Read the model definition and answer for the solid it produces. Units are mm, in the model's axes. A direction names the side the tool comes from. Round coordinates to 2 decimals unless told otherwise and drop trailing zeros. Loops run counter-clockwise (first coordinate to the right, second up) from the corner with the lowest first, then second, coordinate; pieces in that order, holes last. Notation, with made-up numbers: (-16.75, 33) -> (11.25, 33) arc R20 ccw to (11.25, 62) -> close; hole circle Ø5 at (-15, -7.5). An arc over 180 degrees is marked (long way). Put each result on its own line as item: value.
from build123d import *

# Parameters (mm, degrees)
SKETCH_R        = 14
SKETCH_R_2      = 8
PAD_DEPTH       = 2
SKETCH001_R     = 10
SKETCH001_R_2   = 8
PAD001_DEPTH    = 22
CHAMFER_SIZE    = 0.5
CHAMFER001_SIZE = 0.5
CHAMFER002_SIZE = 0.5
CHAMFER003_SIZE = 1


with BuildPart() as part:
    # Sketch → Pad (new body)
    with BuildSketch(Plane.XY):
        Circle(SKETCH_R)
        Circle(SKETCH_R_2, mode=Mode.SUBTRACT)
    extrude(amount=PAD_DEPTH)

    # Sketch001 (on Face4 of Pad) → Pad001 (join)
    with BuildSketch(Plane.XY.offset(2)):
        Circle(SKETCH001_R)
        Circle(SKETCH001_R_2, mode=Mode.SUBTRACT)
    extrude(amount=PAD001_DEPTH)

    # Chamfer
    chamfer_edges = [part.edges().sort_by_distance(p)[0] for p in [
        (-8, 0, 24),
    ]]
    chamfer(chamfer_edges, length=CHAMFER_SIZE)

    # Chamfer001
    chamfer001_edges = [part.edges().sort_by_distance(p)[0] for p in [
        (-10, 0, 24),
    ]]
    chamfer(chamfer001_edges, length=CHAMFER001_SIZE)

    # Chamfer002
    chamfer002_edges = [part.edges().sort_by_distance(p)[0] for p in [
        (-8, 0, 0),
    ]]
    chamfer(chamfer002_edges, length=CHAMFER002_SIZE)

    # Chamfer003
    chamfer003_edges = [part.edges().sort_by_distance(p)[0] for p in [
        (-14, 0, 2),
    ]]
    chamfer(chamfer003_edges, length=CHAMFER003_SIZE)


solid = part.part
Item 1: Flat-ended cylindrical pins translate along their axes: pin 1 Ø4 at (y, z) = (4.5, 21.5) entering from +X; pin 2 Ø4 at (x, z) = (-6, 6) entering from -Y; pin 3 Ø1.5 at (y, z) = (-3.5, 11.5) entering from -X. Find the tip coordinate at first contact, or state that the pin passes through.
Derived:
pin 1: stops at x = 9.68
pin 2: stops at y = -9.17
pin 3: stops at x = -9.61
Item 2: The part is cut by section A-A (x = 0). Determine the outline of the cut face in (y, z), then the cut area to 3 significant figures.
Derived:
outline: (-14, 0) -> (-8.5, 0) -> (-8, 0.5) -> (-8, 23.5) -> (-8.5, 24) -> (-9.5, 24) -> (-10, 23.5) -> (-10, 2) -> (-13, 2) -> (-14, 1) -> close; (8, 0.5) -> (8.5, 0) -> (14, 0) -> (14, 1) -> (13, 2) -> (10, 2) -> (10, 23.5) -> (9.5, 24) -> (8.5, 24) -> (8, 23.5) -> close
area: 110 mm^2
Item 3: Which of the six approach directions +Z, -Z, +X, -X, +Y, -Y give full straight-line access (tool end or side, diameter ignored) to faces 4 (the cylindrical face through (-2.17, -9.76, 12.6)), 5 (the flat face through (0, -9, 0))?
Derived:
face 4: +Z
face 5: -Z, +X, -X, +Y, -Y
Item 4: For a pull along Y with two mould halves and no side action, classify faces 1 (the cylindrical face through (12.932, -5.362, 0.493)), 2 (the flat face through (7, -8, 2)), 3 (the cylindrical face through (-1.73, -7.81, 11.84)) as pulls with the +Y half, pulls with the -Y half, needs draft (parallel to the pull), parting line crosses it, or undercut.
Derived:
face 1: parting line crosses it
face 2: needs draft
face 3: undercut
Item 5: Find the intervals of material crossed by line 1 along Y through (x, z) = (0, 7); line 2 along Y through (x, z) = (-5, 10) (3 decimals); line 3 along X through (y, z) = (5.25, 11), in increasing order.
Derived:
line 1: y = -10 to -8, 8 to 10
line 2: y = -8.66 to -6.245, 6.245 to 8.66
line 3: x = -8.51 to -6.04, 6.04 to 8.51
Item 6: The part is cut by section C-C (z = 19.75). Determine the outline of the cut face in (x, y).
Derived:
outline: circle Ø20 at (0, 0); hole circle Ø16 at (0, 0)
